```python
from build123d import *

# Parameters (mm, degrees)
F1_DEPTH = 25.4
F2_W     = 20.32
F2_H     = 76.557289119
F3_DEPTH = 7.62


with BuildPart() as f1:
    # F0 (on Right) → F1 (new body)
    with BuildSketch(Plane.YZ):
        Polygon((-5.7579418114, 11.3197219973), (0, 0), (67.918331984, 34.5476508683), (62.4788479285, 46.0293610512), align=None)
    extrude(amount=F1_DEPTH)

    # F2 (on face) → F3 (cut)
    with BuildSketch(Plane(origin=(0, -5.7579418114, 11.3197219973), x_dir=(1, 0, 0), z_dir=(0, -0.453381245, 0.8913166927))):
        with Locations((12.7, 38.2786445595)):
            Rectangle(F2_W, F2_H)
    extrude(amount=-F3_DEPTH, mode=Mode.SUBTRACT)


solid = f1.part
```
The model under review builds one solid part; all positions refer to its coordinate system, in mm. A direction names the side the tool comes from. Round coordinates to 2 decimals unless told otherwise and drop trailing zeros. Loops run counter-clockwise (first coordinate to the right, second up) from the corner with the lowest first, then second, coordinate; pieces in that order, holes last. Notation, with made-up numbers: M 37,32 L 92,32 A21 cw 92,52 Z; hole C 29,80.5 d6. An arc over 180 degrees is marked long. Write item = value, one per line.
Item 1: Machinability: for faces 4 (the flat face through (2.54, 30, 25)), 5 (the flat face through (12.52, 33.48, 17.03)), which of the approach directions +Z, -Z, +X, -X, +Y, -Y give a long, thin tool a straight path to every point of the face, cutting with its end or side? Answer none if there is none.
Return value:
face_4 = +Z, -Y
face_5 = -Z, +X, -X, +Y
Item 2: For line 1 (X direction, y = 59, z = 37); line 2 (Y direction, x = 24, z = 22); line 3 (Z direction, x = 16.5, y = 21), list the stretches that pass through material, from the lowest coordinate up. Write a range as [from, to].
Return value:
line_1 = [0, 2.54], [22.86, 25.4]
line_2 = [15.24, 43.25]
line_3 = [10.68, 16.38]
Item 3: The part is to be moulded in two halves that separate along X. For faces 1 (the flat face through (0, 31, 25)), 2 (the flat face through (12.52, -1.64, 3.22)), 3 (the flat face through (22.86, 30, 25)), say which applies: released by +X, released by -X, zero draft, split by the parting line, or undercut.
Return value:
face_1 = released by -X
face_2 = zero draft
face_3 = undercut
Item 4: Insertion check: P1, Ø6, axis at x = 6, z = 19.5, coming from the +Y side; P2, Ø10, axis at x = 14, z = 22.5, coming from the -Y side; P3, Ø4, axis at x = 3.5, y = 40.5, coming from the -Z side; P4, Ø12.5, axis at y = 35.5, z = 26.5, coming from the -X side. Each pin has a flat end and moves straight along its axis. Give the tip position at first contact, or say it passes through.
Return value:
P1 = 44.23
P2 = 23.2
P3 = 19.58
P4 = 0
Item 5: Take a section at B-B on z = 33. Write out the cut boundary in (x, y).
Return value:
outline = M 0,36.86 L 2.54,36.86 L 2.54,53.67 L 22.86,53.67 L 22.86,36.86 L 25.4,36.86 L 25.4,64.88 L 0,64.88 Z
Item 6: Take a section at A-A on y = 24. Write out the cut boundary in (x, z).
Return value:
outline = M 0,12.21 L 25.4,12.21 L 25.4,26.46 L 22.86,26.46 L 22.86,17.91 L 2.54,17.91 L 2.54,26.46 L 0,26.46 Z
Item 7: Take a section at C-C on x = 9. Write out the cut boundary in (y, z), then the cut area to 3 significant figures.
Return value:
outline = M -2.3,4.53 L 0,0 L 67.92,34.55 L 65.74,39.14 Z
area = 387 mm2
